Check sheet for the drawn part. Datum: minimum x, y, z corner. Units: mm. Give positions to 0.01 mm unless a question says otherwise; leave off trailing zeros. Loops run counter-clockwise (first coordinate to the right, second up) from the corner with the lowest first, then second, coordinate; pieces in that order, holes last. Notation, with made-up numbers: M -34.5,41.25 L 0.5,41.25 A20 cw 0.5,57.25 Z; hole C -31.75,-2 d8. An arc over 180 degrees is marked long. Write each question's results on one line, items separated by ' | '. Start each with the question number.
1. Sectioned sample at B-B on y = 108. Record the cut outline in (x, z), and give its area (3 significant figures).
2. Material ranges on line 1 along X through (y, z) = (166.5, 2.25); line 2 along Y through (x, z) = (73.5, 1.95); line 3 along X through (y, z) = (8.5, 2.5), recorded low to high.
3. Go/stop test with flat-tipped pins: pin 1 (1.5 mm diameter, centred on y = 135.5, z = 1.5, fed in from +X); pin 2 (1.6 mm diameter, centred on x = 73.5, y = 166.5, fed in from -Z); pin 3 (0.9 mm diameter, centred on x = 82.5, z = 1.5, fed in from +Y). Record where each tip stops, or that it passes through.
4. Sectioned sample at A-A on z = 1.85. Record the cut outline in (x, y).
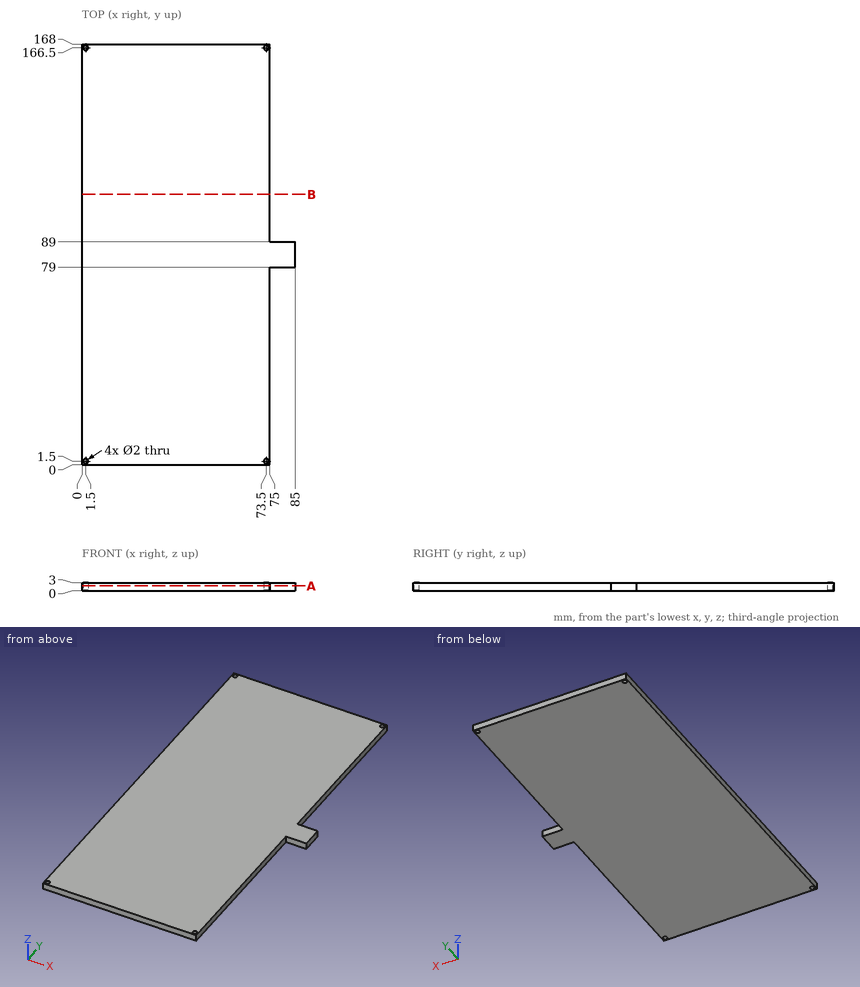
Output values:
1) outline: M 0,0 L 75,0 L 75,3 L 0,3 Z | area: 225 mm2
2) line 1: 0 to 0.5, 2.5 to 72.5, 74.5 to 75 | line 2: 0 to 0.5, 2.5 to 165.5, 167.5 to 168 | line 3: 0 to 75
3) pin 1: x = 75 | pin 2: through | pin 3: y = 89
4) outline: M 0,0 L 75,0 L 75,79 L 85,79 L 85,89 L 75,89 L 75,168 L 0,168 Z; hole C 1.5,1.5 d2; hole C 1.5,166.5 d2; hole C 73.5,1.5 d2; hole C 73.5,166.5 d2
